from build123d import *

# Parameters (mm, degrees)
BOSS_EXTRUDE2_DEPTH = 3


with BuildPart() as part:
    # Sketch1 → Boss-Extrude2 (new body)
    with BuildSketch(Plane(origin=(0, 0, 0), x_dir=(0, 0, -1), z_dir=(1, 0, 0))):
        with BuildLine():
            Line((65, 75), (-65, 75))
            ThreePointArc((-65, 75), (-82.834261673, 64.052022459), (-81.143613719, 43.193911059))
            Line((-81.143613719, 43.193911059), (-32.287227439, -23.612177882))
            ThreePointArc((-32.287227439, -23.612177882), (0, -40), (32.287227439, -23.612177882))
            Line((32.287227439, -23.612177882), (81.143613719, 43.193911059))
            ThreePointArc((81.143613719, 43.193911059), (82.834261673, 64.052022459), (65, 75))
        make_face()
        with BuildLine():
            ThreePointArc((-27.745372612, -11.410271628), (-30, 0), (-27.745372612, 11.410271628))
            ThreePointArc((-27.745372612, 11.410271628), (-29.444863729, 17), (-23.7542714, 18.323061706))
            ThreePointArc((-23.7542714, 18.323061706), (-15, 25.980762114), (-3.991101213, 29.733333333))
            ThreePointArc((-3.991101213, 29.733333333), (-0.133407552, 33.997774684), (4, 30))
            ThreePointArc((4, 30), (3.997774684, 29.866592448), (3.991101213, 29.733333333))
            ThreePointArc((3.991101213, 29.733333333), (15, 25.980762114), (23.7542714, 18.323061706))
            ThreePointArc((23.7542714, 18.323061706), (27.864115127, 18.528878211), (29.980762114, 15))
            ThreePointArc((29.980762114, 15), (29.376232773, 12.885578329), (27.745372612, 11.410271628))
            ThreePointArc((27.745372612, 11.410271628), (30, 0), (27.745372612, -11.410271628))
            ThreePointArc((27.745372612, -11.410271628), (29.376232773, -12.885578329), (29.980762114, -15))
            ThreePointArc((29.980762114, -15), (27.864115127, -18.528878211), (23.7542714, -18.323061706))
            ThreePointArc((23.7542714, -18.323061706), (15, -25.980762114), (3.991101213, -29.733333333))
            ThreePointArc((3.991101213, -29.733333333), (3.997774684, -29.866592448), (4, -30))
            ThreePointArc((4, -30), (-0.133407552, -33.997774684), (-3.991101213, -29.733333333))
            ThreePointArc((-3.991101213, -29.733333333), (-15, -25.980762114), (-23.7542714, -18.323061706))
            ThreePointArc((-23.7542714, -18.323061706), (-29.444863729, -17), (-27.745372612, -11.410271628))
        make_face(mode=Mode.SUBTRACT)
        with BuildLine():
            ThreePointArc((-65, 47), (-73, 55), (-65, 63))
            Line((-65, 63), (-45, 63))
            ThreePointArc((-45, 63), (-37, 55), (-45, 47))
            Line((-45, 47), (-65, 47))
        make_face(mode=Mode.SUBTRACT)
        with BuildLine():
            ThreePointArc((65, 63), (73, 55), (65, 47))
            Line((65, 47), (45, 47))
            ThreePointArc((45, 47), (37, 55), (45, 63))
            Line((45, 63), (65, 63))
        make_face(mode=Mode.SUBTRACT)
    extrude(amount=BOSS_EXTRUDE2_DEPTH)


solid = part.part
Input: part model. Units: mm. Frame: model coordinates. A direction names the side the tool comes from. Give positions to 0.01 mm unless a question says otherwise; leave off trailing zeros. Order: outer loops, then holes, each group sorted by start corner. A loop starts at its lowest first (then second) coordinate and runs counter-clockwise, first axis right, second up. Notation, with made-up numbers: (73, 9) - (93, 9) arc R32 cw to (93, 44) - close; hole circle Ø1 at (20, 32.25). An arc over 180 degrees is marked (long way). Answer as a JSON object with one key per item and string values. Group by question number.
Q1. Cut plane B-B, the plane z = 0. Output: boundary loops of the cut face in (x, y), then the cut area to 3 significant figures.
Q2. First-contact query: pin 1 Ø3 at (y, z) = (37, 38.5) entering from -X. Flat tip, straight axial feed; report the tip coordinate or a pass-through.
Q3. Set-up query: faces 1 (the face through (1.48, 25.9, 15.14)), 2 (the face through (3, 44, 1)). Return all of +Z, -Z, +X, -X, +Y, -Y with unobstructed straight access to the full face (end or side cutting, diameter ignored); none if empty.
Q4. Cut plane C-C, the plane y = 5. Output: boundary loops of the cut face in (x, z), then the cut area to 3 significant figures.
Q5. Line query: probe 1 along Y at (x, z) = (2.4, -26.5); probe 2 along Z at (x, y) = (1, 21); probe 3 along Y at (x, z) = (1.7, -25). Output: solid intervals per line, ascending.
Q6. Cut plane A-A, the plane x = 0.8. Output: boundary loops of the cut face in (y, z).
Q7. Mould query, pull axis Z, two halves, no side actions, for faces 3 (the face through (1.48, 10.26, 57.06)), 4 (the face through (1.48, 63.78, -82.97)), 5 (the face through (1.5, 16.9, 29.5)), 6 (the face through (1.479, -39.997, 0.526)). Classes: pulls with the +Z half, pulls with the -Z half, needs draft (parallel to the pull), parting line crosses it, or undercut.
Results:
{
 "1": {"outline": "(0, -40) - (3, -40) - (3, -34) - (0, -34) - close; (0, 34) - (3, 34) - (3, 75) - (0, 75) - close", "area": "141 mm^2"},
 "2": {"pin 1": "x = 0"},
 "3": {"face 1": "+X, -X", "face 2": "+Z, -Z, +X, +Y, -Y"},
 "4": {"outline": "(0, -53.21) - (3, -53.21) - (3, -29.58) - (0, -29.58) - close; (0, 29.58) - (3, 29.58) - (3, 53.21) - (0, 53.21) - close", "area": "142 mm^2"},
 "5": {"probe 1": "-29.96 to -18.97, 18.97 to 75", "probe 2": "-64.91 to -21.42, 21.42 to 64.91", "probe 3": "-31.22 to -18.88, 18.88 to 75"},
 "6": {"outline": "(-23.61, -32.29) - (43.19, -81.14) arc R20 ccw to (75, -65) - (75, 65) arc R20 ccw to (43.19, 81.14) - (-23.61, 32.29) arc R40 ccw to start; hole (-29.73, -3.99) arc R30 ccw to (-18.32, -23.75) arc R4 ccw (long way) to (-11.41, -27.75) arc R30 ccw to (11.41, -27.75) arc R4 ccw (long way) to (18.32, -23.75) arc R30 ccw to (29.73, -3.99) arc R4 ccw (long way) to (29.73, 3.99) arc R30 ccw to (18.32, 23.75) arc R4 ccw (long way) to (11.41, 27.75) arc R30 ccw to (-11.41, 27.75) arc R4 ccw (long way) to (-18.32, 23.75) arc R30 ccw to (-29.73, 3.99) arc R4 ccw (long way) to start; hole (47, -65) arc R8 ccw to (63, -65) - (63, -45) arc R8 ccw to (47, -45) - close; hole (47, 45) arc R8 ccw to (63, 45) - (63, 65) arc R8 ccw to (47, 65) - close"},
 "7": {"face 3": "pulls with the +Z half", "face 4": "pulls with the -Z half", "face 5": "undercut", "face 6": "parting line crosses it"}
}
